Here's how the part is built. I have some questions about the finished solid (model axes, mm). Face numbers are marked on the shaded views. A direction names the side the tool comes from. Round coordinates to 2 decimals unless told otherwise and drop trailing zeros. Write each loop counter-clockwise with the first axis right and the second up, starting at its lowest first coordinate (ties: lowest second). Pieces come first, ordered by that corner, then holes. Notation, with made-up numbers: (32, 28) -> (81, 28) arc R25 cw to (81, 43) -> close; hole circle Ø11 at (77.25, 81.25). An arc over 180 degrees is marked (long way). Put each result on its own line as item: value. Start each with the question number.
1) We'd pull the mould along X, two halves only. Please class the marked faces 1, 2 and 3: released by +X, released by -X, zero draft, split by the parting line, or undercut.
2) Which directions (+Z, -Z, +X, -X, +Y, -Y) give clear straight access to the entire face, cutting with the end or side of a thin tool? Please do the marked faces 4 and 5.
3) If I drill on line 1 along X through (y, z) = (-24.5, 5.25); line 2 along X through (y, z) = (-6, -0.75); line 3 along Z through (x, y) = (0.5, -15), over which ranges is the centre line in solid material (lowest first)? Write a range as [from, to].
4) I want a section at B-B, the plane y = -10.5. List the corners of the cut face in (x, z) for me.
5) Will these pins go through, and if not, where does the flat tip stop? P1, Ø12, axis at y = 17.5, z = 1, coming from the -X side; P2, Ø12, axis at x = -21, z = -7.5, coming from the -Y side; P3, Ø7.5, axis at x = 15.5, z = 2, coming from the +Y side; P4, Ø4, axis at y = -9, z = -4, coming from the -X side.
6) I want a section at C-C, the plane x = -3.5. List the corners of the cut face in (y, z) for me, then the cut area to 3 significant figures.
7) I want a section at A-A, the plane z = -6. List the corners of the cut face in (x, y) for me, then the cut area to 3 significant figures.
8) I want a section at D-D, the plane y = 20. List the corners of the cut face in (x, z) for me.
from build123d import *

# Parameters (mm, degrees)
F1_DEPTH = 5
F2_DEPTH = 30
F3_R     = 10
F4_DEPTH = 40


with BuildPart() as f1:
    # F0 (on Front) → F1 (new body)
    with BuildSketch(Plane.XZ):
        with BuildLine():
            Line((25, -7.5), (32.5, -7.5))
            Line((32.5, -7.5), (32.5, 0))
            ThreePointArc((32.5, 0), (30.3033008589, -5.3033008589), (25, -7.5))
        make_face()
        with BuildLine():
            Line((-32.5, -7.5), (-25, -7.5))
            ThreePointArc((-25, -7.5), (-30.3033008589, -5.3033008589), (-32.5, 0))
            Line((-32.5, 0), (-32.5, -7.5))
        make_face()
        with BuildLine():
            ThreePointArc((25, 7.5), (30.3033008589, 5.3033008589), (32.5, 0))
            Line((32.5, 0), (32.5, 7.5))
            Line((32.5, 7.5), (25, 7.5))
        make_face()
        with BuildLine():
            Line((-32.5, 7.5), (-32.5, 0))
            ThreePointArc((-32.5, 0), (-30.3033008589, 5.3033008589), (-25, 7.5))
            Line((-25, 7.5), (-32.5, 7.5))
        make_face()
        with BuildLine():
            Line((-25, -7.5), (-2.86e-08, -7.5))
            ThreePointArc((-2.86e-08, -7.5), (-7.5, 1.43e-08), (0, 7.5))
            Line((0, 7.5), (-25, 7.5))
            ThreePointArc((-25, 7.5), (-19.6966991411, 5.3033008589), (-17.5, 0))
            ThreePointArc((-17.5, 0), (-19.6966991411, -5.3033008589), (-25, -7.5))
        make_face()
        with BuildLine():
            ThreePointArc((-32.5, 0), (-30.3033008589, -5.3033008589), (-25, -7.5))
            ThreePointArc((-25, -7.5), (-19.6966991411, -5.3033008589), (-17.5, 0))
            ThreePointArc((-17.5, 0), (-19.6966991411, 5.3033008589), (-25, 7.5))
            ThreePointArc((-25, 7.5), (-30.3033008589, 5.3033008589), (-32.5, 0))
        make_face()
        with BuildLine():
            ThreePointArc((0, 7.5), (-7.5, 1.43e-08), (-2.86e-08, -7.5))
            ThreePointArc((-2.86e-08, -7.5), (5.3033008488, -5.303300869), (7.5, 0))
            ThreePointArc((7.5, 0), (5.3033008589, 5.3033008589), (0, 7.5))
        make_face()
        with BuildLine():
            Line((-2.86e-08, -7.5), (25, -7.5))
            ThreePointArc((25, -7.5), (17.5, 0), (25, 7.5))
            Line((25, 7.5), (0, 7.5))
            ThreePointArc((0, 7.5), (5.3033008589, 5.3033008589), (7.5, 0))
            ThreePointArc((7.5, 0), (5.3033008488, -5.303300869), (-2.86e-08, -7.5))
        make_face()
        with BuildLine():
            ThreePointArc((25, 7.5), (17.5, 0), (25, -7.5))
            ThreePointArc((25, -7.5), (30.3033008589, -5.3033008589), (32.5, 0))
            ThreePointArc((32.5, 0), (30.3033008589, 5.3033008589), (25, 7.5))
        make_face()
    extrude(amount=F1_DEPTH)

    # F0 (on Front) → F2 (join)
    with BuildSketch(Plane.XZ):
        with BuildLine():
            ThreePointArc((-32.5, 0), (-30.3033008589, -5.3033008589), (-25, -7.5))
            ThreePointArc((-25, -7.5), (-19.6966991411, -5.3033008589), (-17.5, 0))
            ThreePointArc((-17.5, 0), (-19.6966991411, 5.3033008589), (-25, 7.5))
            ThreePointArc((-25, 7.5), (-30.3033008589, 5.3033008589), (-32.5, 0))
        make_face()
        with BuildLine():
            ThreePointArc((25, 7.5), (17.5, 0), (25, -7.5))
            ThreePointArc((25, -7.5), (30.3033008589, -5.3033008589), (32.5, 0))
            ThreePointArc((32.5, 0), (30.3033008589, 5.3033008589), (25, 7.5))
        make_face()
        with BuildLine():
            ThreePointArc((0, 7.5), (-7.5, 1.43e-08), (-2.86e-08, -7.5))
            ThreePointArc((-2.86e-08, -7.5), (5.3033008488, -5.303300869), (7.5, 0))
            ThreePointArc((7.5, 0), (5.3033008589, 5.3033008589), (0, 7.5))
        make_face()
    extrude(amount=F2_DEPTH)

    # F3 (on Front) → F4 (join)
    with BuildSketch(Plane.XZ):
        Circle(F3_R)
    extrude(amount=-F4_DEPTH)


solid = f1.part
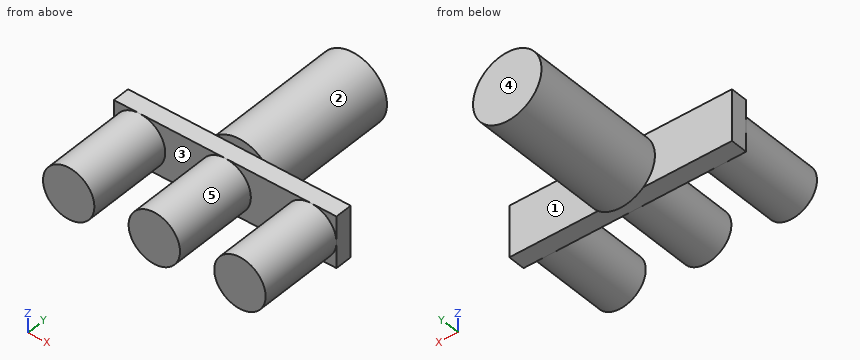
Findings:
1. face 1: zero draft
1. face 2: split by the parting line
1. face 3: undercut
2. face 4: +Z, -Z, +X, -X, +Y
2. face 5: -Y
3. line 1: x = [-30.36, -19.64], [-5.36, 5.36], [19.64, 30.36]
3. line 2: x = [-32.46, -17.54], [-7.46, 7.46], [17.54, 32.46]
3. line 3: z = [-7.48, 7.48]
4. outline: circle Ø15 at (-25, 0); circle Ø15 at (0, 0); circle Ø15 at (25, 0)
5. P1: stops at x = -10
5. P2: stops at y = -30
5. P3: stops at y = 0
5. P4: stops at x = -32.23
6. outline: (-30, -6.63) -> (-5, -6.63) -> (-5, -7.5) -> (0, -7.5) -> (0, -9.37) -> (40, -9.37) -> (40, 9.37) -> (0, 9.37) -> (0, 7.5) -> (-5, 7.5) -> (-5, 6.63) -> (-30, 6.63) -> close
6. area: 1,160 mm2
7. outline: (-32.5, -5) -> (-29.5, -5) -> (-29.5, -30) -> (-20.5, -30) -> (-20.5, -5) -> (-4.5, -5) -> (-4.5, -30) -> (4.5, -30) -> (4.5, -5) -> (20.5, -5) -> (20.5, -30) -> (29.5, -30) -> (29.5, -5) -> (32.5, -5) -> (32.5, 0) -> (8, 0) -> (8, 40) -> (-8, 40) -> (-8, 0) -> (-32.5, 0) -> close
7. area: 1,640 mm2
8. outline: circle Ø20 at (0, 0)
